Could you check a few things on this model? Use its own coordinates, in mm. A direction names the side the tool comes from. Coordinates: 2 decimals unless noted, no trailing zeros. Write each loop counter-clockwise with the first axis right and the second up, starting at its lowest first coordinate (ties: lowest second). Pieces come first, ordered by that corner, then holes.
```python
from build123d import *

# Parameters (mm, degrees)
CUT_EXTRUDE3_DEPTH           = 60
CUT_EXTRUDE5_DEPTH           = 2
CUT_EXTRUDE5_DEPTH_BACK      = 30
SKETCH9_R                    = 38
SKETCH9_R_2                  = 23
SKETCH19_W                   = 12
SKETCH19_H                   = 36.5
CUT_REVOLVE2_ANGLE           = 65
CUT_REVOLVE2_OTHER_WAY_ANGLE = 65
SKETCH21_W                   = 3.25
SKETCH21_H                   = 4
BOSS_EXTRUDE3_DEPTH          = 1.35
CIRPATTERN1_COUNT            = 5
CUT_EXTRUDE9_START           = -5
CUT_EXTRUDE9_DEPTH           = 5
SKETCH23_R                   = 10.5
CUT_EXTRUDE10_DEPTH          = 10
SKETCH24_W                   = 15
SKETCH24_H                   = 8
BOSS_EXTRUDE4_DEPTH          = 8
SKETCH26_W                   = 10
SKETCH26_H                   = 6
CUT_EXTRUDE11_DEPTH          = 10
SKETCH27_W                   = 4
SKETCH27_H                   = 5
CUT_EXTRUDE12_DEPTH          = 5
CUT_EXTRUDE14_DEPTH          = 2
CUT_EXTRUDE14_DEPTH_BACK     = 30
SKETCH29_R                   = 1
CUT_EXTRUDE15_DEPTH          = 15
FILLET1_R                    = 6
FILLET2_R                    = 8
INTERSECT1_DEPTH             = 58.427876097
SKETCH31_W                   = 7
SKETCH31_H                   = 5
BOSS_EXTRUDE7_DEPTH          = 8
SKETCH32_R                   = 1
CUT_EXTRUDE16_DEPTH          = 7.5
FILLET3_R                    = 1


# Read off the part's stored shape, not the designer's step: Cut-Extrude9, Intersect1
with BuildPart() as part:
    # Sketch1 → Revolve1 (revolve)
    with BuildSketch(Plane.XY, mode=Mode.PRIVATE) as revolve1_sk:
        with BuildLine():
            Line((0, 63.427876097), (32, 63.427876097))
            ThreePointArc((32, 63.427876097), (37.656854249, 61.084730346), (40, 55.427876097))
            Line((40, 55.427876097), (40, 28.846818009))
            ThreePointArc((40, 28.846818009), (38.792081772, 24.082439968), (35.460140376, 20.469057744))
            Line((35.460140376, 20.469057744), (28.539859624, 15.958818353))
            ThreePointArc((28.539859624, 15.958818353), (25.207918228, 12.345436129), (24, 7.581058088))
            Line((24, 7.581058088), (24, 3.25))
            Line((24, 3.25), (24.35, 3))
            Line((24.35, 3), (24.35, 0))
            Line((24.35, 0), (22.5, 0))
            Line((22.5, 0), (22.5, 12.5))
            ThreePointArc((22.5, 12.5), (22.353553391, 12.853553391), (22, 13))
            Line((22, 13), (0, 13))
            Line((0, 13), (0, 63.427876097))
        make_face()
    revolve(revolve1_sk.sketch.rotate(Axis((0, 0, 0), (0, 1, 0)), 90), axis=Axis((0, 0, 0), (0, 1, 0)))

    # Sketch11 → Cut-Extrude3 (cut)
    with BuildSketch(Plane(origin=(0, 13, 0), x_dir=(-1, 0, 0), z_dir=(0, -1, 0))):
        with BuildLine():
            Line((-21, 0), (21, 0))
            ThreePointArc((21, 0), (0, 21), (-21, 0))
        make_face()
    extrude(amount=-CUT_EXTRUDE3_DEPTH, mode=Mode.SUBTRACT)

    # Sketch9 → Cut-Extrude5 (cut, two sides: drawn at the far end of the back side and taken through both)
    with BuildSketch(Plane(origin=(0, 55.427876097, 0), x_dir=(1, 0, 0), z_dir=(0, 1, 0)).offset(-CUT_EXTRUDE5_DEPTH_BACK)):
        with Locations(Location((0, 0, 0), (0, 0, 270))):
            Circle(SKETCH9_R)
        with Locations(Location((0, 0, 0), (0, 0, 270))):
            Circle(SKETCH9_R_2, mode=Mode.SUBTRACT)
    extrude(amount=CUT_EXTRUDE5_DEPTH + CUT_EXTRUDE5_DEPTH_BACK, mode=Mode.SUBTRACT)

    # Sketch19 → Cut-Revolve2 (revolve, cut)
    with BuildSketch(Plane(origin=(0, 0, 0), x_dir=(0, 0, -1), z_dir=(1, 0, 0))):
        with Locations((-41.064715832, 37.177876097)):
            Rectangle(SKETCH19_W, SKETCH19_H)
    revolve(axis=Axis((0, 0, 0), (0, 1, 0)), revolution_arc=CUT_REVOLVE2_ANGLE, mode=Mode.SUBTRACT)

    # Sketch19 → Cut-Revolve2 other way (revolve, cut)
    with BuildSketch(Plane(origin=(0, 0, 0), x_dir=(0, 0, -1), z_dir=(1, 0, 0))):
        with Locations((-41.064715832, 37.177876097)):
            Rectangle(SKETCH19_W, SKETCH19_H)
    revolve(axis=Axis((0, 0, 0), (0, -1, 0)), revolution_arc=CUT_REVOLVE2_OTHER_WAY_ANGLE, mode=Mode.SUBTRACT)

    # Sketch21 → Boss-Extrude3 (add)
    with BuildSketch(Plane(origin=(0, 0, 22.5), x_dir=(-1, 0, 0), z_dir=(0, 0, -1))):
        with Locations((0, 2)):
            Rectangle(SKETCH21_W, SKETCH21_H)
    boss_extrude3 = extrude(amount=BOSS_EXTRUDE3_DEPTH)

    # CirPattern1: Boss-Extrude3 ×5 about axis
    cirpattern1_axis = Axis((0, 0, 0), (0, 1, 0))
    for i in range(1, CIRPATTERN1_COUNT):
        add(boss_extrude3.rotate(cirpattern1_axis, i * 360 / CIRPATTERN1_COUNT))

    # Cut-Extrude9 outline → Cut-Extrude9 (cut)
    with BuildSketch(Plane(origin=(0, 63.427876097, 0), x_dir=(1, 0, 0), z_dir=(0, 1, 0)).offset(CUT_EXTRUDE9_START)):
        with BuildLine():
            ThreePointArc((40, 0), (0, 40), (-40, 0))
            Line((-40, 0), (-21, 0))
            ThreePointArc((-21, 0), (0, 21), (21, 0))
            Line((21, 0), (40, 0))
        make_face()
    extrude(amount=CUT_EXTRUDE9_DEPTH, mode=Mode.SUBTRACT)

    # Sketch23 → Cut-Extrude10 (cut)
    with BuildSketch(Plane(origin=(0, 0, -40), x_dir=(-1, 0, 0), z_dir=(0, 0, -1))):
        with Locations((0, 42.137876097)):
            Circle(SKETCH23_R)
    extrude(amount=-CUT_EXTRUDE10_DEPTH, mode=Mode.SUBTRACT)

    # Sketch24 → Boss-Extrude4 (add)
    with BuildSketch(Plane(origin=(0, 58.427876097, 0), x_dir=(1, 0, 0), z_dir=(0, 1, 0))):
        with Locations((0, 30)):
            Rectangle(SKETCH24_W, SKETCH24_H)
    extrude(amount=-BOSS_EXTRUDE4_DEPTH)

    # Sketch26 → Cut-Extrude11 (cut)
    with BuildSketch(Plane(origin=(0, 58.427876097, 0), x_dir=(1, 0, 0), z_dir=(0, 1, 0))):
        with Locations((0, 30)):
            Rectangle(SKETCH26_W, SKETCH26_H)
    extrude(amount=-CUT_EXTRUDE11_DEPTH, mode=Mode.SUBTRACT)

    # Sketch27 → Cut-Extrude12 (cut)
    with BuildSketch(Plane(origin=(7.5, 0, 0), x_dir=(0, 0, -1), z_dir=(1, 0, 0))):
        with Locations((30, 53.927876097)):
            Rectangle(SKETCH27_W, SKETCH27_H)
    extrude(amount=-CUT_EXTRUDE12_DEPTH, mode=Mode.SUBTRACT)

    # Sketch28 → Cut-Extrude14 (cut, two sides: drawn at the far end of the back side and taken through both)
    with BuildSketch(Plane(origin=(0, 55.427876097, 0), x_dir=(1, 0, 0), z_dir=(0, 1, 0)).offset(-CUT_EXTRUDE14_DEPTH_BACK)):
        with BuildLine():
            Line((-22.912878475, -2), (22.912878475, -2))
            ThreePointArc((22.912878475, -2), (0, -23), (-22.912878475, -2))
        make_face()
    extrude(amount=CUT_EXTRUDE14_DEPTH + CUT_EXTRUDE14_DEPTH_BACK, mode=Mode.SUBTRACT)

    # Sketch29 → Cut-Extrude15 (cut)
    with BuildSketch(Plane(origin=(0, 0, 0), x_dir=(-1, 0, 0), z_dir=(0, 0, -1))):
        with Locations((-30.416198487, 60.927876097)):
            Circle(SKETCH29_R)
        with Locations((30.416198487, 60.927876097)):
            Circle(SKETCH29_R)
        with Locations((0, 60.927876097)):
            Circle(SKETCH29_R)
    extrude(amount=-CUT_EXTRUDE15_DEPTH, mode=Mode.SUBTRACT)

    # Fillet1
    fillet1_edges = [part.edges().sort_by_distance(p)[0] for p in [
        (21, 35.713938048, 0),
        (-21, 35.713938048, 0),
    ]]
    fillet(fillet1_edges, radius=FILLET1_R)

    # Fillet2
    fillet2_edges = [part.edges().sort_by_distance(p)[0] for p in [
        (-22.912878475, 41.427876097, 2),
        (22.912878475, 41.427876097, 2),
    ]]
    fillet(fillet2_edges, radius=FILLET2_R)

    # Intersect1 outline → Intersect1 (cut)
    with BuildSketch(Plane(origin=(0, 0, 0), x_dir=(1, 0, 0), z_dir=(0, 1, 0))):
        with BuildLine():
            Line((-37.508702776, -13.895942431), (-42, -15.355253362))
            Line((-42, -15.355253362), (-42, -41))
            Line((-42, -41), (42, -41))
            Line((42, -41), (42, -15.355253362))
            Line((42, -15.355253362), (37.508702776, -13.895942431))
            ThreePointArc((37.508702776, -13.895942431), (0, 40), (-37.508702776, -13.895942431))
        make_face()
        with BuildLine():
            ThreePointArc((19.246817919, 8.4), (18.767687244, 2.713664655), (13.747727085, 0))
            Line((13.747727085, 0), (-13.747727085, 0))
            ThreePointArc((-13.747727085, 0), (-18.767687244, 2.713664655), (-19.246817919, 8.4))
            ThreePointArc((-19.246817919, 8.4), (0, 21), (19.246817919, 8.4))
        make_face(mode=Mode.SUBTRACT)
    extrude(amount=INTERSECT1_DEPTH, mode=Mode.SUBTRACT)

    # Sketch31 → Boss-Extrude7 (add)
    with BuildSketch(Plane(origin=(0, 58.427876097, 0), x_dir=(1, 0, 0), z_dir=(0, 1, 0))):
        with Locations((0, -29.5)):
            Rectangle(SKETCH31_W, SKETCH31_H)
    extrude(amount=-BOSS_EXTRUDE7_DEPTH)

    # Sketch32 → Cut-Extrude16 (cut)
    with BuildSketch(Plane(origin=(3.5, 0, 0), x_dir=(0, 0, -1), z_dir=(1, 0, 0))):
        with Locations((-29.5, 54.427876097)):
            Circle(SKETCH32_R)
    extrude(amount=-CUT_EXTRUDE16_DEPTH, mode=Mode.SUBTRACT)

    # Fillet3
    fillet3_edges = [part.edges().sort_by_distance(p)[0] for p in [
        (0, 58.427876097, 0),
    ]]
    fillet(fillet3_edges, radius=FILLET3_R)


solid = part.part
```
Item 1: I want a section at B-B, the plane y = 56.25. List the corners of the cut face in (x, z) for me, then the cut area to 3 significant figures.
Item 2: I want a section at A-A, the plane x = 0. List the corners of the cut face in (y, z) for me.
Item 3: If we mould it in two halves opening along Z, with no side actions, what happens to faces 1 (the flat face through (1, 62, 0)), 2 (the cylindrical face through (0.049, 53.452, 29.717)), 3 (the cylindrical face through (30.63, 59.95, 7.4))? For each: released by +Z, released by -Z, zero draft, split by the parting line, or undercut.
Item 4: Which directions (+Z, -Z, +X, -X, +Y, -Y) give clear straight access to the entire face, cutting with the end or side of a thin tool? Please do faces 4 (the flat face through (0, 54, 27)), 5 (the flat face through (0, 61, 15)), 6 (the flat face through (3.5, 54, 31)).
Item 5: If I drill on line 1 along Y through (x, z) = (-1, 29.5); line 2 along Y through (x, z) = (17, 18); line 3 along X through (y, z) = (60.5, 4.5), over which ranges is the centre line in solid material (lowest first)?
Item 6: Will these pins go through, and if not, where does the flat tip stop? pin 1 Ø5.5 at (x, y) = (1.5, 53.5) entering from +Z; pin 2 Ø1.6 at (x, y) = (-30.5, 61) entering from -Z; pin 3 Ø5.5 at (y, z) = (56, 29) entering from +X.
Item 7: I want a section at C-C, the plane z = 12.5. Count the separate pieces of the cut face and the enclosed holes in it, then the cut area to 3 significant figures.
Taken from the geometry:
1. outline: (-3.5, 27) - (3.5, 27) - (3.5, 32) - (-3.5, 32) - close
1. area: 35.0 mm2
2. outline: (50.43, 27) - (58.43, 27) - (58.43, 1) arc R1 ccw to (59.43, 0) - (59.93, 0) - (59.93, 15) - (61.93, 15) - (61.93, 0) - (63.43, 0) - (63.43, 32) arc R8 ccw to (58.43, 39.42) - (58.43, 32) - (50.43, 32) - close; hole circle Ø2 at (54.43, 29.5)
3. face 1: released by -Z
3. face 2: undercut
3. face 3: zero draft
4. face 4: -Z, +X, -X, -Y
4. face 5: -Z
4. face 6: +Z, -Z, +X, -Y
5. line 1: y = 50.43 to 53.43, 55.43 to 63.43
5. line 2: y = 58.43 to 63.43
5. line 3: x = -37.92 to -31.32, -29.51 to -0.9, 0.9 to 29.51, 31.32 to 37.92
6. pin 1: stops at z = 32
6. pin 2: stops at z = 15
6. pin 3: stops at x = 28.03
7. separate pieces: 1
7. enclosed holes: 3
7. area: 343 mm2
